The listing builds one solid part. Answer for the finished solid, in the listing's coordinates (mm). Round coordinates to 2 decimals unless told otherwise and drop trailing zeros. Loops run counter-clockwise (first coordinate to the right, second up) from the corner with the lowest first, then second, coordinate; pieces in that order, holes last. Notation, with made-up numbers: (13, -34) -> (53, -34) arc R14 cw to (53, -20) -> close; hole circle Ø1 at (48, 51.25). An arc over 180 degrees is marked (long way). One line per question, with ' | ' between items.
from build123d import *

# Parameters (mm, degrees)
CROQUIS1_R                 = 1.5
SALIENTE_EXTRUIR1_DEPTH    = 3
S_LIDO_MOVER_COPIAR1_ANGLE = 90


with BuildPart() as part:
    # Croquis1 → Saliente-Extruir1 (new body)
    with BuildSketch(Plane.XY):
        with BuildLine():
            Line((41840.173257962, -436.939495492), (41840.173257962, -351.939495492))
            ThreePointArc((41840.173257962, -351.939495492), (41836.173257962, -347.939495492), (41832.173257962, -351.939495492))
            Line((41832.173257962, -351.939495492), (41832.173257962, -436.939495492))
            Line((41832.173257962, -436.939495492), (41832.173257962, -438.939495492))
            ThreePointArc((41832.173257962, -438.939495492), (41836.173257962, -442.939495492), (41840.173257962, -438.939495492))
            Line((41840.173257962, -438.939495492), (41840.173257962, -436.939495492))
        make_face()
        with Locations((41836.173257962, -351.939495492)):
            Circle(CROQUIS1_R, mode=Mode.SUBTRACT)
        with Locations((41836.173257962, -438.939495492)):
            Circle(CROQUIS1_R, mode=Mode.SUBTRACT)
    extrude(amount=SALIENTE_EXTRUIR1_DEPTH)


with BuildPart() as part_1:
    # Sólido-Mover/Copiar1: moved
    add(part.part.rotate(Axis((0, -394.439495492, 1.5), (1, 0, 0)), S_LIDO_MOVER_COPIAR1_ANGLE))


solid = part_1.part
Q1. Find the intervals of material crossed by line 1 (Z direction, x = 41836, y = -393.5); line 2 (X direction, y = -394.5, z = -43); line 3 (Z direction, x = 41837, y = -393.8), in increasing order. Write a range as from..to.
Numbers:
line 1: -47..-44.49, -41.51..42.51, 45.49..48 | line 2: 41832.17..41834.67, 41837.67..41840.17 | line 3: -46.91..-44.25, -41.75..42.75, 45.25..47.91
Q2. For a pull along X with two mould halves and no side action, classify faces 1 (the face through (41837.56, -394.42, -43.57)), 2 (the face through (41836, -392.939, 1)), 3 (the face through (41836.1, -394.4, -47)) as pulls with the +X half, pulls with the -X half, needs draft (parallel to the pull), parting line crosses it, or undercut.
Numbers:
face 1: undercut | face 2: needs draft | face 3: parting line crosses it
Q3. A cutting plane is placed at A-A on y = -394.05. Give the vertices of the cut face in (x, z), plus the area to 3 significant figures.
Numbers:
outline: (41832.17, -43) arc R4 ccw to (41840.17, -43) -> (41840.17, 44) arc R4 ccw to (41832.17, 44) -> close; hole circle Ø3 at (41836.17, -43); hole circle Ø3 at (41836.17, 44) | area: 732 mm^2
Q4. A cutting plane is placed at B-B on x = 41838.5. Give the vertices of the cut face in (y, z), plus the area to 3 significant figures.
Numbers:
outline: (-395.94, -46.25) -> (-392.94, -46.25) -> (-392.94, 47.25) -> (-395.94, 47.25) -> close | area: 281 mm^2
